from build123d import *

# Parameters (mm, degrees)
SKETCH_1_R          = 30
EXTRUDE_1_DEPTH     = 70
EXTRUDE_START       = 43
SKETCH_1_4_R        = 7.5
EXTRUDE_2_DEPTH     = 15
SKETCH_3_R          = 20
CUT_EXTRUDE_1_DEPTH = 15
CUT_EXTRUDE_2_DEPTH = 91.277350426


with BuildPart() as part:
    # Sketch 1 → Extrude 1 (new body)
    with BuildSketch(Plane(origin=(0, 0, 0), x_dir=(1, 0, 0), z_dir=(0, 1, 0))):
        with Locations(Location((0, 0, 0), (0, 0, 270))):
            Circle(SKETCH_1_R)
    extrude(amount=EXTRUDE_1_DEPTH)

    # Sketch 1_4 → Extrude 2 (add)
    with BuildSketch(Plane(origin=(0, 0, 0), x_dir=(1, 0, 0), z_dir=(0, 1, 0)).offset(EXTRUDE_START)):
        with BuildLine():
            ThreePointArc((25.980762114, 15), (30, 0), (25.980762114, -15))
            Line((25.980762114, -15), (50, -15))
            ThreePointArc((50, -15), (65, 0), (50, 15))
            Line((50, 15), (25.980762114, 15))
        make_face()
        with Locations(Location((50, 0, 0), (0, 0, 270))):
            Circle(SKETCH_1_4_R, mode=Mode.SUBTRACT)
    extrude(amount=EXTRUDE_2_DEPTH)

    # Sketch 3 → Cut-Extrude 1 (cut)
    with BuildSketch(Plane(origin=(0, 70, 0), x_dir=(1, 0, 0), z_dir=(0, 1, 0))):
        with Locations(Location((0, 0, 0), (0, 0, 270))):
            Circle(SKETCH_3_R)
    extrude(amount=-CUT_EXTRUDE_1_DEPTH, mode=Mode.SUBTRACT)

    # Sketch 4 → Cut-Extrude 2 (cut, through all)
    with BuildSketch(Plane(origin=(0, 55, 0), x_dir=(1, 0, 0), z_dir=(0, 1, 0))):
        Polygon((0, -12.727922061), (-12.727922061, 0), (0, 12.727922061), (12.727922061, 0), align=None)
    extrude(amount=-CUT_EXTRUDE_2_DEPTH, mode=Mode.SUBTRACT)


solid = part.part
Geometry check sheet. Reference: the model listing, model coordinates, mm. A direction names the side the tool comes from. Round coordinates to 2 decimals unless told otherwise and drop trailing zeros. Loops run counter-clockwise (first coordinate to the right, second up) from the corner with the lowest first, then second, coordinate; pieces in that order, holes last. Notation, with made-up numbers: (25, 88) -> (84, 88) arc R23 ccw to (84, 120) -> close; hole circle Ø10 at (66, -30). An arc over 180 degrees is marked (long way). Answer as a JSON object with one key per item and string values. Group by question number.
Item 1: Set-up check for faces 1 (the face through (7, 0, 6)), 2 (the face through (-4, 55, 9)), 3 (the face through (6.453, 27.885, 6.275)): record each of +Z, -Z, +X, -X, +Y, -Y from which the full face is reachable in a straight line by a thin tool's end or side.
Item 2: Depth check by flat-ended pin: pin 1 Ø7.5 at (x, y) = (36.5, 52) entering from +Z; pin 2 Ø12 at (x, y) = (7, 56.5) entering from -Z; pin 3 Ø3 at (y, z) = (51.5, 23.5) entering from -X. Enter the tip coordinate at first touch or a pass-through.
Item 3: Release check for a two-part mould opening along Z. For faces 4 (the face through (-6.275, 27.885, 6.453)), 5 (the face through (38, 50, 15)), 6 (the face through (41, 43, 0)), 7 (the face through (38, 50, -15)) record: pulls with the +Z half, pulls with the -Z half, needs draft (parallel to the pull), parting line crosses it, or undercut.
Item 4: Cross-section at B-B, the plane x = 47. Record the cut outline in (y, z).
Item 5: Cross-section at A-A, the plane z = -5. Record the cut outline in (x, y).
Item 6: Thickness scan on line 1 along X through (y, z) = (54, 0); line 2 along X through (y, z) = (63.25, 0); line 3 along Z through (x, y) = (47, 51.5). Record the ranges inside material, lowest first.
Item 7: Cross-section at D-D, the plane x = 14.5. Record the cut outline in (y, z), plus the area to 3 significant figures.
Item 8: Cross-section at C-C, the plane y = 15. Record the cut outline in (x, z), plus the area to 3 significant figures.
Determined:
{
 "1": {"face 1": "+Z, -Z, +X, -X, -Y", "face 2": "+Y", "face 3": "+Y, -Y"},
 "2": {"pin 1": "stops at z = 15", "pin 2": "stops at z = -29.98", "pin 3": "stops at x = -20.4"},
 "3": {"face 4": "undercut", "face 5": "pulls with the +Z half", "face 6": "needs draft", "face 7": "pulls with the -Z half"},
 "4": {"outline": "(43, -15) -> (58, -15) -> (58, -6.87) -> (43, -6.87) -> close; (43, 6.87) -> (58, 6.87) -> (58, 15) -> (43, 15) -> close"},
 "5": {"outline": "(-29.58, 0) -> (-7.73, 0) -> (-7.73, 55) -> (-19.36, 55) -> (-19.36, 70) -> (-29.58, 70) -> close; (7.73, 0) -> (29.58, 0) -> (29.58, 43) -> (44.41, 43) -> (44.41, 58) -> (29.58, 58) -> (29.58, 70) -> (19.36, 70) -> (19.36, 55) -> (7.73, 55) -> close; (55.59, 43) -> (64.14, 43) -> (64.14, 58) -> (55.59, 58) -> close"},
 "6": {"line 1": "x = -30 to -12.73, 12.73 to 42.5, 57.5 to 65", "line 2": "x = -30 to -20, 20 to 30", "line 3": "z = -15 to -6.87, 6.87 to 15"},
 "7": {"outline": "(0, -26.26) -> (70, -26.26) -> (70, -13.77) -> (55, -13.77) -> (55, 13.77) -> (70, 13.77) -> (70, 26.26) -> (0, 26.26) -> close", "area": "3,260 mm²"},
 "8": {"outline": "circle Ø60 at (0, 0); hole (-12.73, 0) -> (0, -12.73) -> (12.73, 0) -> (0, 12.73) -> close", "area": "2,500 mm²"}
}
